Build history of the part. All positions in model axes, mm. Face numbers are marked on the shaded views. A direction names the side the tool comes from. Give positions to 0.01 mm unless a question says otherwise; leave off trailing zeros. Order: outer loops, then holes, each group sorted by start corner. A loop starts at its lowest first (then second) coordinate and runs counter-clockwise, first axis right, second up. Notation, with made-up numbers: (-4, -28) - (15, -28) arc R22 cw to (15, -22) - close; hole circle Ø7 at (-34, -38). An arc over 180 degrees is marked (long way). Use a Markdown table: item, result. Add a question column.
(1) Slice it at B-B (x = 37.5). Write the cut outline in (y, z).
(2) Wall check: line 1 (Z direction, x = -29, y = -10); line 2 (X direction, y = -1, z = 70); line 3 (X direction, y = 16, z = 42.5). Give the ranges that are in metal, low to high.
(3) Which spindle directions (+Z, -Z, +X, -X, +Y, -Y) get a long thin tool onto all of the face, cutting with end or side? Do the marked faces 1 and 2. Say none if no direction does.
(4) Slice it at C-C (z = 61). Write the cut outline in (x, y), then the cut area to 3 significant figures.
(5) Slice it at A-A (y = 0). Write the cut outline in (x, z), then the cut area to 3 significant figures.
(6) Flat gauge pins, fed straight in: pin 1 (12 mm diameter, centred on y = -8, z = 32, fed in from -X) (3 decimals); pin 2 (5 mm diameter, centred on y = -21, z = 45.5, fed in from +X); pin 3 (10 mm diameter, centred on y = 14.5, z = 42, fed in from +X). Where does each tip first touch, or does it go through?
(7) Slice it at D-D (y = -17.5). Write the cut outline in (x, z), then the cut area to 3 significant figures.
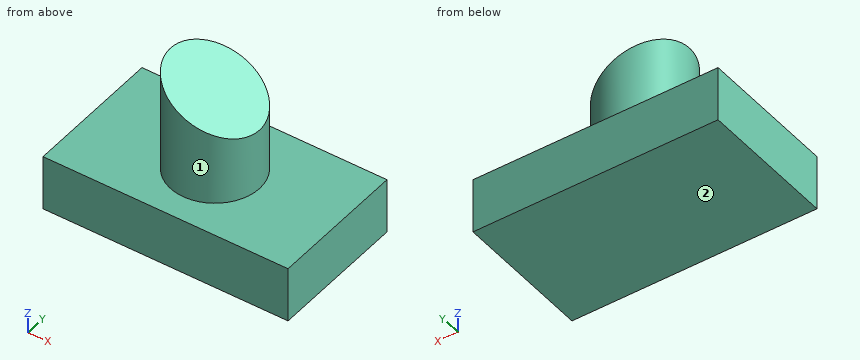
from build123d import *

# Parameters (mm, degrees)
F0_W     = 112.405978
F0_H     = 63.648052
F1_DEPTH = 25.4
F2_R     = 20.433121
F3_DEPTH = 50.8
F5_DEPTH = 25.4


with BuildPart() as f1:
    # F0 (on Top) → F1 (new body)
    with BuildSketch(Plane.XY):
        Rectangle(F0_W, F0_H)
    extrude(amount=F1_DEPTH)

    # F2 (on face) → F3 (join)
    with BuildSketch(Plane.XY.offset(25.4)):
        Circle(F2_R)
    extrude(amount=F3_DEPTH)

    # F4 (on Front) → F5 (cut, symmetric)
    with BuildSketch(Plane.XZ):
        Polygon((42.320769, 80.948107), (-34.6261, 80.948107), (42.320769, 43.09025), align=None)
    extrude(amount=F5_DEPTH, both=True, mode=Mode.SUBTRACT)


solid = f1.part
Solution:
| question | item | result |
|---|---|---|
| 1 | outline | (-31.82, 0) - (31.82, 0) - (31.82, 25.4) - (-31.82, 25.4) - close |
| 2 | line 1 | 0 to 25.4 |
| 2 | line 2 | -20.41 to -12.37 |
| 2 | line 3 | -12.71 to 12.71 |
| 3 | face 1 | +Z |
| 3 | face 2 | -Z, +X, -X, +Y, -Y |
| 4 | outline | (5.92, -19.56) - (5.92, 19.56) arc R20.43 ccw (long way) to start |
| 4 | area | 894 mm2 |
| 5 | outline | (-56.2, 0) - (56.2, 0) - (56.2, 25.4) - (20.43, 25.4) - (20.43, 53.86) - (-20.43, 73.97) - (-20.43, 25.4) - (-56.2, 25.4) - close |
| 5 | area | 4,430 mm2 |
| 6 | pin 1 | x = -20.335 |
| 6 | pin 2 | x = 8.68 |
| 6 | pin 3 | x = 18.09 |
| 7 | outline | (-56.2, 0) - (56.2, 0) - (56.2, 25.4) - (10.55, 25.4) - (10.55, 58.72) - (-10.55, 69.1) - (-10.55, 25.4) - (-56.2, 25.4) - close |
| 7 | area | 3,670 mm2 |
